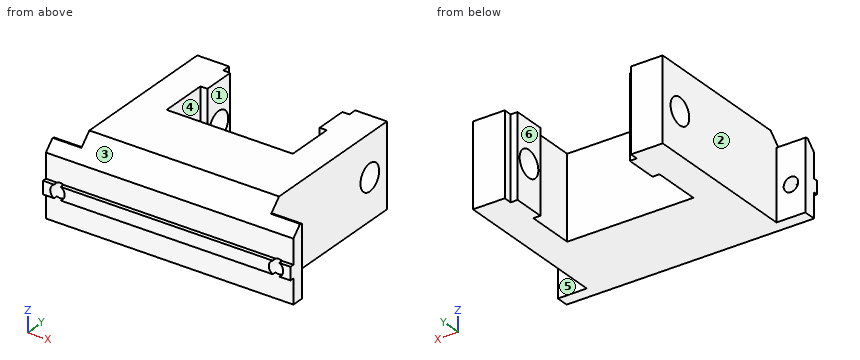
Autodesk Fusion 360 part; units mm, degrees
sketch "Sketch1" plane through (0, 0, 0) normal (0, 0, 1) x (1, 0, 0)
  line L0 (0, 0) -> (46, 0)
  line L1 (46, 0) -> (46, 20.6)
  line L2 (46, 20.6) -> (0, 20.6)
  line L3 (0, 20.6) -> (0, 0)
  line L4 (0, 20.6) -> (7.7, 20.6)
  line L5 (7.7, 20.6) -> (7.7, 40)
  line L6 (7.7, 40) -> (0, 40)
  line L7 (0, 40) -> (0, 20.6)
  line L8 (7.7, 40) -> (9.4, 40)
  line L9 (9.4, 40) -> (9.4, 32.2)
  line L10 (9.4, 32.2) -> (7.7, 32.2)
  line L11 (7.7, 32.2) -> (7.7, 40)
  line L12 (23, 20.6) -> (23, 0) construction
  line L13 (46, 20.6) -> (38.3, 20.6)
  line L14 (38.3, 20.6) -> (38.3, 40)
  line L15 (46, 40) -> (46, 20.6)
  line L16 (38.3, 40) -> (46, 40)
  line L17 (38.3, 40) -> (36.6, 40)
  line L18 (36.6, 32.2) -> (38.3, 32.2)
  line L19 (38.3, 32.2) -> (38.3, 40)
  line L20 (36.6, 40) -> (36.6, 32.2)
  line L21 (0, 0) -> (-7, 0)
  line L22 (-7, 0) -> (-7, 3)
  line L23 (-7, 3) -> (0, 3)
  line L24 (0, 3) -> (0, 0)
  line L25 (46, 0) -> (53, 0)
  line L26 (53, 0) -> (53, 3)
  line L27 (53, 3) -> (46, 3)
  line L28 (46, 3) -> (46, 0)
  dimension "d1" = 20.6
  dimension "d2" = 46
  dimension "d3" = 7.7
  dimension "d6" = 40
  dimension "d7" = 7.8
  dimension "d8" = 1.7
  dimension "d9" = 7
  dimension "d10" = 3
  dimension "d11" = 3
  dimension "d12" = 7
extrude "Extrude1" add sketch "Sketch1" along normal blind 20
chamfer "Chamfer1" distance 5 angle 45 1 edges at (23, 0, 20)
sketch "Sketch2" plane through (-7, 0, 0) normal (-1, 0, 0) x (0, 0, 1)
  line L0 (15, 0) -> (18, 3)
  line L1 (18, 3) -> (0, 3)
  line L2 (0, 3) -> (0, 0)
  line L3 (0, 0) -> (15, 0)
  line L4 (5.95, 0) -> (9.05, 0)
  line L5 (9.05, 0) -> (9.05, -1)
  line L6 (9.05, -1) -> (5.95, -1)
  line L7 (5.95, -1) -> (5.95, 0)
  point P0 (7.5, 0)
  dimension "d16" = 1
  dimension "d17" = 3.1
extrude "Extrude2" add sketch "Sketch2" against normal up to surface (60 mm away) contours L3 L4 L5 L6 L7
sketch "Sketch3" plane through (0, 0, 0) normal (-1, 0, 0) x (0, 0, 1)
  line L0 (18, 3) -> (20, 5)
  line L1 (20, 5) -> (20, 40)
  line L2 (20, 40) -> (0, 40)
  line L3 (0, 40) -> (0, 3)
  line L4 (0, 3) -> (18, 3)
  circle A0 centre (10, 36.1) radius 3.2
  line L5 (0, 40) -> (0, 32.2)
  point P0 (10, 40)
  point P1 (0, 36.1)
  dimension "d20" = 6.4
extrude "Extrude3" cut sketch "Sketch3" against normal through all contours A0
sketch "Sketch4" plane through (0, 40, 0) normal (0, 1, 0) x (-1, 0, 0)
  line L0 (-9.4, 0) -> (0, 0)
  line L1 (0, 0) -> (0, 20)
  line L2 (0, 20) -> (-9.4, 20)
  line L3 (-9.4, 20) -> (-9.4, 0)
  line L4 (0, 0) -> (-7.7, 0)
  line L5 (-7.7, 0) -> (-7.7, 20)
  line L6 (-7.7, 20) -> (0, 20)
  line L7 (0, 20) -> (0, 0)
  point P0 (-7.7, 0)
extrude "Extrude4" add sketch "Sketch4" along normal blind 2 contours L0 L1 L2 L4 L5 L6 L7
ref_plane "WorkPlane1" through (23, 22.5, 10) normal (-1, 0, 0) x (0, -1, 0)
mirror "Mirror1" about plane through (23, 22.5, 10) normal (-1, 0, 0) of "Extrude4"
sketch "Sketch5" plane through (0, 3, 0) normal (0, 1, 0) x (-1, 0, 0)
  line L0 (7, 18) -> (0, 18)
  line L1 (0, 18) -> (0, 0)
  line L2 (0, 0) -> (7, 0)
  line L3 (7, 0) -> (7, 18)
  line L4 (7, 9.05) -> (7, 5.95)
  circle A0 centre (3.5, 7.5) radius 1.75
  point P0 (7, 7.5)
  dimension "d25" = 3.5
  dimension "d26" = 3.5
extrude "Extrude5" cut sketch "Sketch5" against normal blind 5 contours A0
mirror "Mirror2" about plane through (23, 22.5, 10) normal (-1, 0, 0) of "Extrude5"
chamfer "Chamfer2" distance 1 angle 45 2 edges at (49.5, 3, 18) (-3.5, 3, 18)
equation "d11 = d10"
equation "d12 = d9"
Source: CAD feature listing. Evaluate the final solid. Frame: model axes, mm. Face numbers are marked on the shaded views. A direction names the side the tool comes from. Give positions to 0.01 mm unless a question says otherwise; leave off trailing zeros. Write each loop counter-clockwise with the first axis right and the second up, starting at its lowest first coordinate (ties: lowest second). Pieces come first, ordered by that corner, then holes.
1. Section query C-C (x = -3.5). Return the cut outline in (y, z).
2. Material intervals for line 1 along X through (y, z) = (2.2, 7.5); line 2 along Y through (x, z) = (5.25, 10); line 3 along Z through (x, y) = (38, 36), sorted ascending.
3. Section query A-A (y = 27.5). Return the cut outline in (x, z).
4. Section query D-D (y = 36.1). Return the cut outline in (x, z).
5. Access query for the marked faces 4, 5 and 6. Directions: +Z, -Z, +X, -X, +Y, -Y. A direction counts if a zero-diameter tool reaches every point of the face in a straight line with its end or side. Return the directions, or none.
6. Section query B-B (z = 10). Return the cut outline in (x, y), then the cut area to 3 significant figures.
7. Pull-direction query (X, two-part tool) for the marked faces 1, 2 and 3; classes: +X half, -X half, draft (parallel to the pull), parting line (faces both ways), or undercut.
8. First-contact query: pin 1 (5.5 mm diameter, centred on x = 50, z = 5, fed in from +Y); pin 2 (2 mm diameter, centred on y = 41, z = 13, fed in from -X); pin 3 (0.5 mm diameter, centred on x = 8.5, z = 6.5, fed in from +Y). Flat tips, straight axial feed; report the tip coordinate or a pass-through.
Output values:
1. outline: (0, 0) - (3, 0) - (3, 5.75) - (0, 5.75) - close; (0, 9.25) - (3, 9.25) - (3, 17) - (2.29, 17.29) - (0, 15) - close
2. line 1: x = -7 to -5.25, -1.75 to 47.75, 51.25 to 53
2. line 2: y = 0 to 32.9, 39.3 to 42
2. line 3: z = 0 to 6.8, 13.2 to 20
3. outline: (0, 0) - (7.7, 0) - (7.7, 20) - (0, 20) - close; (38.3, 0) - (46, 0) - (46, 20) - (38.3, 20) - close
4. outline: (0, 0) - (9.4, 0) - (9.4, 6.8) - (0, 6.8) - close; (0, 13.2) - (9.4, 13.2) - (9.4, 20) - (0, 20) - close; (36.6, 0) - (46, 0) - (46, 6.8) - (36.6, 6.8) - close; (36.6, 13.2) - (46, 13.2) - (46, 20) - (36.6, 20) - close
5. face 4: +Z, -Z
5. face 5: +Z, -Z, +X, +Y
5. face 6: +Z, -Z, +Y
6. outline: (-7, 0) - (53, 0) - (53, 3) - (46, 3) - (46, 32.9) - (36.6, 32.9) - (36.6, 32.2) - (38.3, 32.2) - (38.3, 20.6) - (7.7, 20.6) - (7.7, 32.2) - (9.4, 32.2) - (9.4, 32.9) - (0, 32.9) - (0, 3) - (-7, 3) - close; (0, 39.3) - (9.4, 39.3) - (9.4, 40) - (7.7, 40) - (7.7, 42) - (0, 42) - close; (36.6, 39.3) - (46, 39.3) - (46, 42) - (38.3, 42) - (38.3, 40) - (36.6, 40) - close
6. area: 1,230 mm2
7. face 1: undercut
7. face 2: -X half
7. face 3: draft
8. pin 1: stops at y = 3
8. pin 2: stops at x = 0
8. pin 3: stops at y = 40
